Input: dimensioned drawing with shaded views. Units: mm. Origin: part minimum x, y, z. A direction names the side the tool comes from. Coordinates: 2 decimals unless noted, no trailing zeros. Order: outer loops, then holes, each group sorted by start corner. A loop starts at its lowest first (then second) coordinate and runs counter-clockwise, first axis right, second up. Notation, with made-up numbers: (86.5, -21.5) - (129.5, -21.5) arc R11 ccw to (129.5, -16.5) - close; hole circle Ø4 at (46, -6.5). An arc over 180 degrees is marked (long way). Answer as CSV lines item,"result". Start each with the question number.
Item 1: Draft query along Y for the marked faces 1, 2, 3 and 4. Return one class per face: +Y half, -Y half, draft (parallel to the pull), parting line (faces both ways), or undercut.
Item 2: First-contact query: pin 1 (5.5 mm diameter, centred on x = 33.5, z = 2, fed in from +Y); pin 2 (3 mm diameter, centred on x = 37, y = 7.5, fed in from +Z); pin 3 (1.5 mm diameter, centred on x = 20, z = 2.5, fed in from -Y). Flat tips, straight axial feed; report the tip coordinate or a pass-through.
Item 3: Section B-B (x = 55). Output: boundary loops of the cut face in (y, z), and give its area (3 significant figures).
Item 4: Section D-D (z = 7.25). Output: boundary loops of the cut face in (x, y), and give its area (3 significant figures).
Item 5: Access query for the marked faces 5 and 6. Directions: +Z, -Z, +X, -X, +Y, -Y. A direction counts if a zero-diameter tool reaches every point of the face in a straight line with its end or side. Return the directions, or none.
Item 6: Section A-A (z = 1.75). Output: boundary loops of the cut face in (x, y).
Item 7: Material intervals for line 1 along Y through (x, z) = (5, 5); line 2 along Z through (x, y) = (35, 5.75); line 3 along Y through (x, z) = (13.5, 2), sorted ascending.
Item 8: Section C-C (x = 9). Output: boundary loops of the cut face in (y, z).
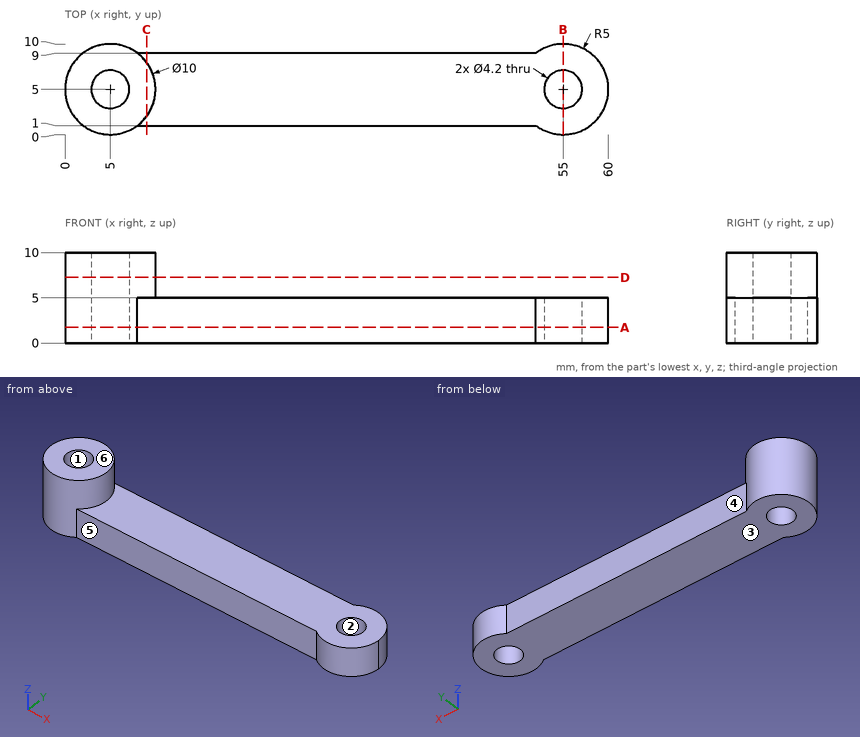
Determined:
1,face 1,"undercut"
1,face 2,"undercut"
1,face 3,"draft"
1,face 4,"+Y half"
2,pin 1,"stops at y = 9"
2,pin 2,"stops at z = 5"
2,pin 3,"stops at y = 1"
3,outline,"(0, 0) - (2.9, 0) - (2.9, 5) - (0, 5) - close; (7.1, 0) - (10, 0) - (10, 5) - (7.1, 5) - close"
3,area,"29.0 mm^2"
4,outline,"circle Ø10 at (5, 5); hole circle Ø4.2 at (5, 5)"
4,area,"64.7 mm^2"
5,face 5,"+Z, -Z, -Y"
5,face 6,"+Z, +X, -X, +Y, -Y"
6,outline,"(8, 1) - (52, 1) arc R5 ccw (long way) to (52, 9) - (8, 9) arc R5 ccw (long way) to start; hole circle Ø4.2 at (5, 5); hole circle Ø4.2 at (55, 5)"
7,line 1,"y = 0 to 2.9, 7.1 to 10"
7,line 2,"z = 0 to 5"
7,line 3,"y = 1 to 9"
8,outline,"(1, 0) - (9, 0) - (9, 5) - (8, 5) - (8, 10) - (2, 10) - (2, 5) - (1, 5) - close"
